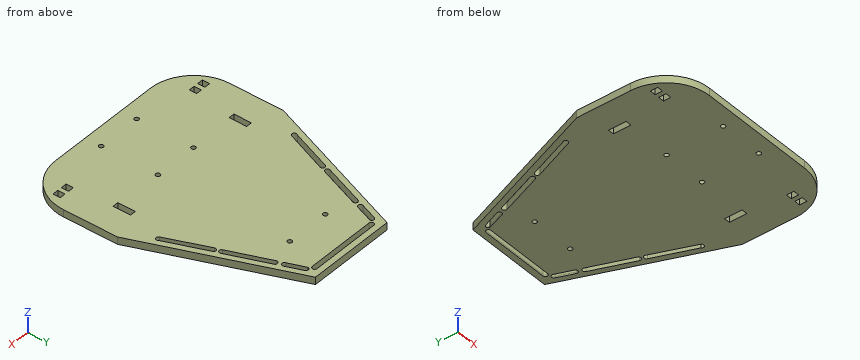
from build123d import *

# Parameters (mm, degrees)
BOSS_EXTRUDE2_DEPTH  = 1
SKETCH41_W           = 4
SKETCH41_H           = 5
SKETCH41_R           = 1.5
SKETCH41_H_2         = 12
CUT_EXTRUDE42_DEPTH  = 19
BOSS_EXTRUDE17_DEPTH = 4
SKETCH47_W           = 4
SKETCH47_H           = 5
SKETCH47_H_2         = 12
CUT_EXTRUDE47_DEPTH  = 185.495850796
SKETCH48_R           = 1.5
CUT_EXTRUDE44_DEPTH  = 185.495850796
BOSS_EXTRUDE18_START = -1
SKETCH51_R           = 1.5
BOSS_EXTRUDE18_DEPTH = 1
BOSS_EXTRUDE19_START = -2
SKETCH52_R           = 1.5
BOSS_EXTRUDE19_DEPTH = 2
SKETCH53_R           = 1.5
CUT_EXTRUDE46_DEPTH  = 185.495850796
BOSS_EXTRUDE20_START = -1
SKETCH55_R           = 1.5
BOSS_EXTRUDE20_DEPTH = 1
SKETCH58_R           = 1.5
CUT_EXTRUDE45_DEPTH  = 185.495850796


with BuildPart() as part:
    # Sketch2 → Boss-Extrude2 (new body)
    with BuildSketch(Plane.XY):
        with BuildLine():
            Line((0, 0), (40, 0))
            ThreePointArc((40, 0), (61.213203436, 8.786796564), (70, 30))
            Line((70, 30), (70, 67))
            Line((70, 67), (30.2211576, 170.627427341))
            Line((30.2211576, 170.627427341), (-30.2211576, 170.627427341))
            Line((-30.2211576, 170.627427341), (-70, 67))
            Line((-70, 67), (-70, 30))
            ThreePointArc((-70, 30), (-61.213203436, 8.786796564), (-40, 0))
            Line((-40, 0), (0, 0))
        make_face()
    extrude(amount=BOSS_EXTRUDE2_DEPTH)

    # Sketch41 → Cut-Extrude42 (cut)
    with BuildSketch(Plane.XY.offset(1)):
        with Locations((54.037011669, 19.5)):
            Rectangle(SKETCH41_W, SKETCH41_H)
        with Locations((-54.037011669, 19.5)):
            Rectangle(SKETCH41_W, SKETCH41_H)
        with Locations((-15, 65)):
            Circle(SKETCH41_R)
        with Locations((15, 65)):
            Circle(SKETCH41_R)
        with BuildLine():
            ThreePointArc((-55.895620015, 84.257333662), (-58.330916289, 83.551440528), (-58.390755847, 86.086272335))
            Line((-58.390755847, 86.086272335), (-47.63971736, 114.09368513))
            ThreePointArc((-47.63971736, 114.09368513), (-45.555710052, 115.00290606), (-44.646489123, 112.918898752))
            Line((-44.646489123, 112.918898752), (-55.895620015, 84.257333662))
        make_face()
        with BuildLine():
            ThreePointArc((-43.178836535, 117.313137537), (-45.24430647, 116.38910618), (-46.168337826, 118.454576116))
            Line((-46.168337826, 118.454576116), (-35.46735115, 146.481150722))
            ThreePointArc((-35.46735115, 146.481150722), (-33.401881215, 147.405182078), (-32.477849859, 145.339712143))
            Line((-32.477849859, 145.339712143), (-43.178836535, 117.313137537))
        make_face()
        with BuildLine():
            ThreePointArc((24, 166.627427341), (25.6, 165.027427341), (24, 163.427427341))
            Line((24, 163.427427341), (-24, 163.427427341))
            ThreePointArc((-24, 163.427427341), (-25.6, 165.027427341), (-24, 166.627427341))
            Line((-24, 166.627427341), (24, 166.627427341))
        make_face()
        with BuildLine():
            ThreePointArc((33.563613753, 151.467161805), (32.441986519, 149.340557263), (30.477844504, 150.727150454))
            Line((30.477844504, 150.727150454), (26.188468437, 162.107072358))
            ThreePointArc((26.188468437, 162.107072358), (27.498296965, 163.680540031), (29.283219083, 162.677791648))
            Line((29.283219083, 162.677791648), (33.563613753, 151.467161805))
        make_face()
        with BuildLine():
            Line((55.895620015, 84.257333662), (44.646489123, 112.918898752))
            ThreePointArc((44.646489123, 112.918898752), (45.555710052, 115.00290606), (47.63971736, 114.09368513))
            Line((47.63971736, 114.09368513), (58.390755847, 86.086272335))
            ThreePointArc((58.390755847, 86.086272335), (58.330916289, 83.551440528), (55.895620015, 84.257333662))
        make_face()
        with Locations((-15, 140.627427341)):
            Circle(SKETCH41_R)
        with Locations((15, 140.627427341)):
            Circle(SKETCH41_R)
        with Locations((49, 54.5)):
            Rectangle(SKETCH41_W, SKETCH41_H_2)
        with Locations((-49, 54.5)):
            Rectangle(SKETCH41_W, SKETCH41_H_2)
        with Locations((61.037011669, 19.5)):
            Rectangle(SKETCH41_W, SKETCH41_H)
        with Locations(Location((15, 15, 0), (0, 0, 180))):
            Circle(SKETCH41_R)
        with Locations((-15, 15)):
            Circle(SKETCH41_R)
        with Locations((-61.037011669, 19.5)):
            Rectangle(SKETCH41_W, SKETCH41_H)
        with BuildLine():
            Line((-33.563613753, 151.467161805), (-29.283219083, 162.677791648))
            ThreePointArc((-29.283219083, 162.677791648), (-27.498296965, 163.680540031), (-26.188468437, 162.107072358))
            Line((-26.188468437, 162.107072358), (-30.477844504, 150.727150454))
            ThreePointArc((-30.477844504, 150.727150454), (-32.441986519, 149.340557263), (-33.563613753, 151.467161805))
        make_face()
        with BuildLine():
            Line((35.46735115, 146.481150722), (46.168337826, 118.454576116))
            ThreePointArc((46.168337826, 118.454576116), (45.24430647, 116.38910618), (43.178836535, 117.313137537))
            Line((43.178836535, 117.313137537), (32.477849859, 145.339712143))
            ThreePointArc((32.477849859, 145.339712143), (33.401881215, 147.405182078), (35.46735115, 146.481150722))
        make_face()
    extrude(amount=-CUT_EXTRUDE42_DEPTH, mode=Mode.SUBTRACT)

    # Sketch42 → Boss-Extrude17 (add)
    with BuildSketch(Plane.XY.offset(1)):
        with BuildLine():
            Line((-40, 0), (40, 0))
            ThreePointArc((40, 0), (61.213203436, 8.786796564), (70, 30))
            Line((70, 30), (70, 67))
            Line((70, 67), (30.2211576, 170.627427341))
            Line((30.2211576, 170.627427341), (-30.2211576, 170.627427341))
            Line((-30.2211576, 170.627427341), (-70, 67))
            Line((-70, 67), (-70, 30))
            ThreePointArc((-70, 30), (-61.213203436, 8.786796564), (-40, 0))
        make_face()
    extrude(amount=BOSS_EXTRUDE17_DEPTH)

    # Sketch47 → Cut-Extrude47 (cut, through all)
    with BuildSketch(Plane(origin=(0, 0, 0), x_dir=(-1, 0, 0), z_dir=(0, 0, -1))):
        with Locations((61.037011669, 19.5)):
            Rectangle(SKETCH47_W, SKETCH47_H)
        with Locations((54.037011669, 19.5)):
            Rectangle(SKETCH47_W, SKETCH47_H)
        with Locations((-54.037011669, 19.5)):
            Rectangle(SKETCH47_W, SKETCH47_H)
        with Locations((-61.037011669, 19.5)):
            Rectangle(SKETCH47_W, SKETCH47_H)
        with Locations((-49, 54.5)):
            Rectangle(SKETCH47_W, SKETCH47_H_2)
        with Locations((49, 54.5)):
            Rectangle(SKETCH47_W, SKETCH47_H_2)
    extrude(amount=-CUT_EXTRUDE47_DEPTH, mode=Mode.SUBTRACT)

    # Sketch48 → Cut-Extrude44 (cut, through all)
    with BuildSketch(Plane(origin=(0, 0, 0), x_dir=(-1, 0, 0), z_dir=(0, 0, -1))):
        with Locations((-15, 140.627427341)):
            Circle(SKETCH48_R)
        with Locations((15, 140.627427341)):
            Circle(SKETCH48_R)
        with BuildLine():
            Line((-43.178836535, 117.313137537), (-32.477849859, 145.339712143))
            ThreePointArc((-32.477849859, 145.339712143), (-33.401881215, 147.405182078), (-35.46735115, 146.481150722))
            Line((-35.46735115, 146.481150722), (-46.168337826, 118.454576116))
            ThreePointArc((-46.168337826, 118.454576116), (-45.24430647, 116.38910618), (-43.178836535, 117.313137537))
        make_face()
        with BuildLine():
            Line((-55.895620015, 84.257333662), (-44.646489123, 112.918898752))
            ThreePointArc((-44.646489123, 112.918898752), (-45.555710052, 115.00290606), (-47.63971736, 114.09368513))
            Line((-47.63971736, 114.09368513), (-58.390755847, 86.086272335))
            ThreePointArc((-58.390755847, 86.086272335), (-58.330916289, 83.551440528), (-55.895620015, 84.257333662))
        make_face()
        with BuildLine():
            Line((-30.477844504, 150.727150454), (-26.188468437, 162.107072358))
            ThreePointArc((-26.188468437, 162.107072358), (-27.498296965, 163.680540031), (-29.283219083, 162.677791648))
            Line((-29.283219083, 162.677791648), (-33.563613753, 151.467161805))
            ThreePointArc((-33.563613753, 151.467161805), (-32.441986519, 149.340557263), (-30.477844504, 150.727150454))
        make_face()
        with BuildLine():
            Line((-24, 163.427427341), (24, 163.427427341))
            ThreePointArc((24, 163.427427341), (25.6, 165.027427341), (24, 166.627427341))
            Line((24, 166.627427341), (-24, 166.627427341))
            ThreePointArc((-24, 166.627427341), (-25.6, 165.027427341), (-24, 163.427427341))
        make_face()
        with BuildLine():
            Line((26.188468437, 162.107072358), (30.477844504, 150.727150454))
            ThreePointArc((30.477844504, 150.727150454), (32.441986519, 149.340557263), (33.563613753, 151.467161805))
            Line((33.563613753, 151.467161805), (29.283219083, 162.677791648))
            ThreePointArc((29.283219083, 162.677791648), (27.498296965, 163.680540031), (26.188468437, 162.107072358))
        make_face()
        with BuildLine():
            Line((46.168337826, 118.454576116), (35.46735115, 146.481150722))
            ThreePointArc((35.46735115, 146.481150722), (33.401881215, 147.405182078), (32.477849859, 145.339712143))
            Line((32.477849859, 145.339712143), (43.178836535, 117.313137537))
            ThreePointArc((43.178836535, 117.313137537), (45.24430647, 116.38910618), (46.168337826, 118.454576116))
        make_face()
        with BuildLine():
            Line((58.390755847, 86.086272335), (47.63971736, 114.09368513))
            ThreePointArc((47.63971736, 114.09368513), (45.555710052, 115.00290606), (44.646489123, 112.918898752))
            Line((44.646489123, 112.918898752), (55.895620015, 84.257333662))
            ThreePointArc((55.895620015, 84.257333662), (58.330916289, 83.551440528), (58.390755847, 86.086272335))
        make_face()
    extrude(amount=-CUT_EXTRUDE44_DEPTH, mode=Mode.SUBTRACT)

    # Sketch51 → Boss-Extrude18 (add)
    with BuildSketch(Plane(origin=(0, 0, 0), x_dir=(-1, 0, 0), z_dir=(0, 0, -1)).offset(BOSS_EXTRUDE18_START)):
        with Locations((-15, 65)):
            Circle(SKETCH51_R)
    extrude(amount=BOSS_EXTRUDE18_DEPTH)

    # Sketch52 → Boss-Extrude19 (add)
    with BuildSketch(Plane(origin=(0, 0, 0), x_dir=(-1, 0, 0), z_dir=(0, 0, -1)).offset(BOSS_EXTRUDE19_START)):
        with Locations((15, 65)):
            Circle(SKETCH52_R)
    extrude(amount=BOSS_EXTRUDE19_DEPTH)

    # Sketch53 → Cut-Extrude46 (cut, through all)
    with BuildSketch(Plane.XY.offset(5)):
        with Locations((-15, 50)):
            Circle(SKETCH53_R)
        with Locations((15, 50)):
            Circle(SKETCH53_R)
    extrude(amount=-CUT_EXTRUDE46_DEPTH, mode=Mode.SUBTRACT)

    # Sketch55 → Boss-Extrude20 (add)
    with BuildSketch(Plane(origin=(0, 0, 0), x_dir=(-1, 0, 0), z_dir=(0, 0, -1)).offset(BOSS_EXTRUDE20_START)):
        with Locations((-15, 15)):
            Circle(SKETCH55_R)
        with Locations((15, 15)):
            Circle(SKETCH55_R)
    extrude(amount=BOSS_EXTRUDE20_DEPTH)

    # Sketch58 → Cut-Extrude45 (cut, through all)
    with BuildSketch(Plane(origin=(0, 0, 0), x_dir=(-1, 0, 0), z_dir=(0, 0, -1))):
        with Locations((-15, 11)):
            Circle(SKETCH58_R)
        with Locations((15, 11)):
            Circle(SKETCH58_R)
    extrude(amount=-CUT_EXTRUDE45_DEPTH, mode=Mode.SUBTRACT)


solid = part.part
The model under review builds one solid part; all positions refer to its coordinate system, in mm. Coordinates: 2 decimals unless noted, no trailing zeros. Write each loop counter-clockwise with the first axis right and the second up, starting at its lowest first coordinate (ties: lowest second). Pieces come first, ordered by that corner, then holes. Notation, with made-up numbers: (-27, 32.5) -> (18, 32.5) arc R27 ccw to (18, 63.5) -> close; hole circle Ø7 at (-18.75, 88.25). An arc over 180 degrees is marked (long way). Answer in a Markdown table with one row per item.
1. We need section B-B, the plane y = 155. State the section outline as (x, z) points, and give its area (3 significant figures).
Answers below:
| item | result |
|---|---|
| outline | (-36.22, 0) -> (-32.21, 0) -> (-32.21, 5) -> (-36.22, 5) -> close; (-28.87, 0) -> (28.87, 0) -> (28.87, 5) -> (-28.87, 5) -> close; (32.21, 0) -> (36.22, 0) -> (36.22, 5) -> (32.21, 5) -> close |
| area | 329 mm^2 |
2. We need section D-D, the plane y = 131.5. State the section outline as (x, z) points, and give its area (3 significant figures).
Answers below:
| item | result |
|---|---|
| outline | (-45.24, 0) -> (-41.19, 0) -> (-41.19, 5) -> (-45.24, 5) -> close; (-37.76, 0) -> (37.76, 0) -> (37.76, 5) -> (-37.76, 5) -> close; (41.19, 0) -> (45.24, 0) -> (45.24, 5) -> (41.19, 5) -> close |
| area | 418 mm^2 |
3. We need section C-C, the plane z = 2.3. Give the number of separate pieces and of enclosed holes in the cut face, and give its area (3 significant figures).
Answers below:
| item | result |
|---|---|
| separate pieces | 1 |
| enclosed holes | 19 |
| area | 18,500 mm^2 |
4. We need section A-A, the plane x = 8.5. State the section outline as (y, z) points.
Answers below:
| item | result |
|---|---|
| outline | (0, 0) -> (163.43, 0) -> (163.43, 5) -> (0, 5) -> close; (166.63, 0) -> (170.63, 0) -> (170.63, 5) -> (166.63, 5) -> close |
5. Clearance check with flat-ended pins moving along their axes: pin 1 Ø2.5 at (y, z) = (19.5, 3.5) entering from +X; pin 2 Ø2 at (y, z) = (100, 3.5) entering from -X; pin 3 Ø1.5 at (y, z) = (20.5, 2) entering from -X. State where each tip first meets the part, or that it passes through.
Answers below:
| item | result |
|---|---|
| pin 1 | stops at x = 68.54 |
| pin 2 | stops at x = -57.72 |
| pin 3 | stops at x = -68.7 |
6. Wall thickness on probe 1 along Y at (x, z) = (-15, 3.8); probe 2 along Y at (x, z) = (19, 4.55); probe 3 along X at (y, z) = (55, 3.75): over which ranges is each line inside the solid? List them lowest first. Write a range as [from, to].
Answers below:
| item | result |
|---|---|
| probe 1 | y = [0, 9.5], [12.5, 48.5], [51.5, 139.13], [142.13, 163.43], [166.63, 170.63] |
| probe 2 | y = [0, 163.43], [166.63, 170.63] |
| probe 3 | x = [-70, -51], [-47, 47], [51, 70] |
